Design review of the part shown in the three views and the two pictorial views. Dimensions are in mm from the part's minimum x, y and z. Give positions to 0.01 mm unless a question says otherwise; leave off trailing zeros. Loops run counter-clockwise (first coordinate to the right, second up) from the corner with the lowest first, then second, coordinate; pieces in that order, holes last.
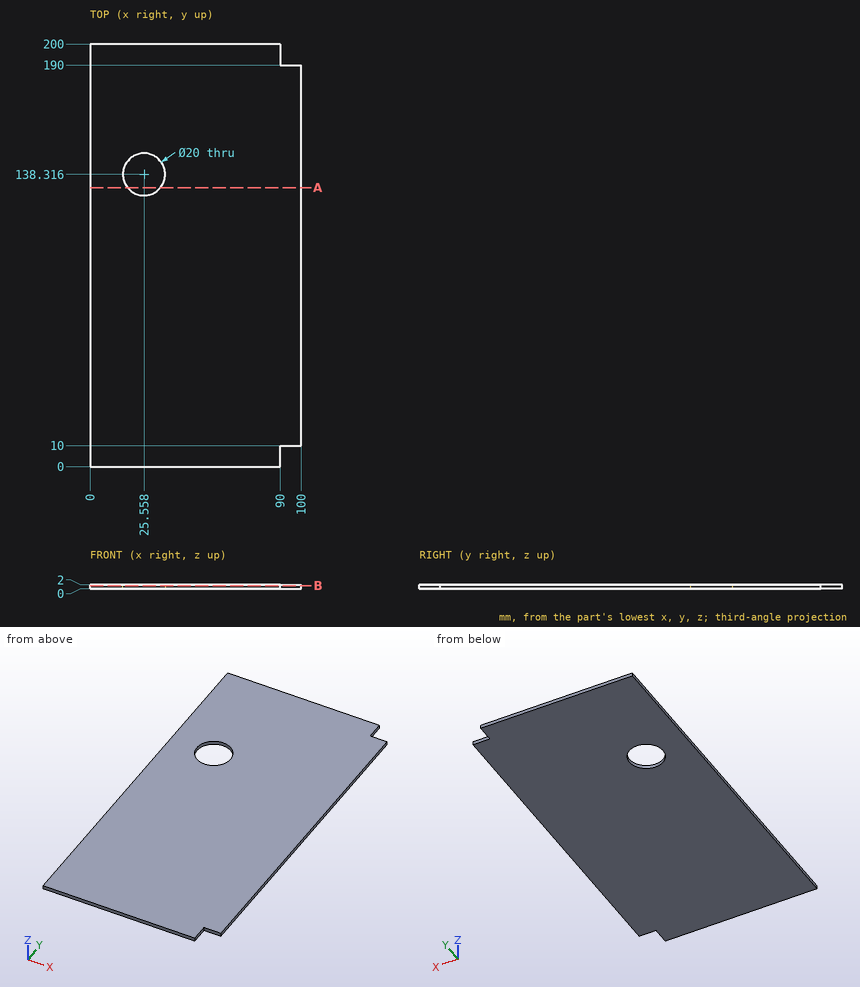
Q1. Take a section at A-A (y = 132). Give the boundary of the cut face in (x, z) (1 decimal).
Results:
outline: (0, 0) - (17.8, 0) - (17.8, 2) - (0, 2) - close; (33.3, 0) - (100, 0) - (100, 2) - (33.3, 2) - close
Q2. Insertion check: pin 1 (1 mm diameter, centred on x = 28.5, y = 24.5, fed in from -Z); pin 2 (18 mm diameter, centred on x = 25.56, y = 138.32, fed in from +Z); pin 3 (0.6 mm diameter, centred on x = 94.5, z = 0.5, fed in from +Y); pin 4 (0.6 mm diameter, centred on x = 94.5, z = 1, fed in from -Y). Each pin has a flat end and moves straight along its axis. Give the tip position at first contact, or say it passes through.
Results:
pin 1: stops at z = 0
pin 2: passes through
pin 3: stops at y = 190
pin 4: stops at y = 10
Q3. Wall thickness on line 1 (Y direction, x = 95, z = 1.8); line 2 (Y direction, x = 33.5, z = 1.5); line 3 (X direction, y = 9, z = 1.6): over which ranges is each line inside the solid? List them lowest first.
Results:
line 1: y = 10 to 190
line 2: y = 0 to 132.24, 144.39 to 200
line 3: x = 0 to 90
Q4. Take a section at B-B (z = 1.55). Give the boundary of the cut face in (x, y).
Results:
outline: (0, 0) - (90, 0) - (90, 10) - (100, 10) - (100, 190) - (90, 190) - (90, 200) - (0, 200) - close; hole circle Ø20 at (25.56, 138.32)
